The listing builds one solid part. Answer for the finished solid, in the listing's coordinates (mm). Coordinates: 2 decimals unless noted, no trailing zeros. Order: outer loops, then holes, each group sorted by start corner. A loop starts at its lowest first (then second) coordinate and runs counter-clockwise, first axis right, second up. Notation, with made-up numbers: M 24,22 L 41,22 A10 cw 41,35 Z; hole C -6.5,68 d3. An arc over 180 degrees is marked long. One line per item, written item: value. Start each with the question number.
Q1. The part is cut by section A-A on y = 4.45. Give the vertices of the cut face in (x, z), then the cut area to 3 significant figures.
Q2. Straight lines are drawn through the part: line 1 along X through (y, z) = (3.05, -53.5); line 2 along Z through (x, y) = (99, 3); line 3 along X through (y, z) = (5.15, -38). For each, find the intervals that lie inside material, in ascending order. Write a range as [from, to].
Q3. Each of these flat-tipped pins is pushed along its axis until it touches: pin 1 Ø10 at (x, z) = (42, -93) entering from -Y; pin 2 Ø1.7 at (y, z) = (2, -87) entering from -X; pin 3 Ø1 at (y, z) = (1.5, -30) entering from +X. Where does it stop, or does it pass through?
Q4. The part is cut by section B-B on z = -87. Give the vertices of the cut face in (x, y).
```python
from build123d import *

# Parameters (mm, degrees)
SKETCH3_W           = 192
SKETCH3_H           = 135
BOSS_EXTRUDE1_DEPTH = 5.7
SKETCH11_R          = 0.5
CUT_EXTRUDE2_DEPTH  = 33
CUT_EXTRUDE3_DEPTH  = 22


with BuildPart() as part:
    # Sketch3 → Boss-Extrude1 (new body)
    with BuildSketch(Plane(origin=(0, 0, 0), x_dir=(1, 0, 0), z_dir=(0, 1, 0))):
        with Locations((90, 53.5)):
            Rectangle(SKETCH3_W, SKETCH3_H)
    extrude(amount=BOSS_EXTRUDE1_DEPTH)

    # Sketch11 → Cut-Extrude2 (cut)
    with BuildSketch(Plane(origin=(0, 0, 0), x_dir=(1, 0, 0), z_dir=(0, 1, 0))):
        with Locations((99, 53.5)):
            Circle(SKETCH11_R)
        with Locations((154.2, 53.5)):
            Circle(SKETCH11_R)
    extrude(amount=CUT_EXTRUDE2_DEPTH, mode=Mode.SUBTRACT)

    # Sketch12 → Cut-Extrude3 (cut)
    with BuildSketch(Plane(origin=(0, 0, 0), x_dir=(1, 0, 0), z_dir=(0, 1, 0))):
        Polygon((-5.8, 121), (-5.8, 93.9), (0, 93.9), (0, 67.1), (-5.8, 67.1), (-5.8, 39.9), (0, 39.9), (0, 13.1), (-5.8, 13.1), (-5.8, -14), (-9.8, -14), (-9.8, 121), align=None)
        Polygon((189.8, 121), (185.8, 121), (185.8, 93.9), (180, 93.9), (180, 67.1), (185.8, 67.1), (185.8, 39.9), (180, 39.9), (180, 13.1), (185.8, 13.1), (185.8, -14), (189.8, -14), align=None)
    extrude(amount=CUT_EXTRUDE3_DEPTH, mode=Mode.SUBTRACT)


solid = part.part
```
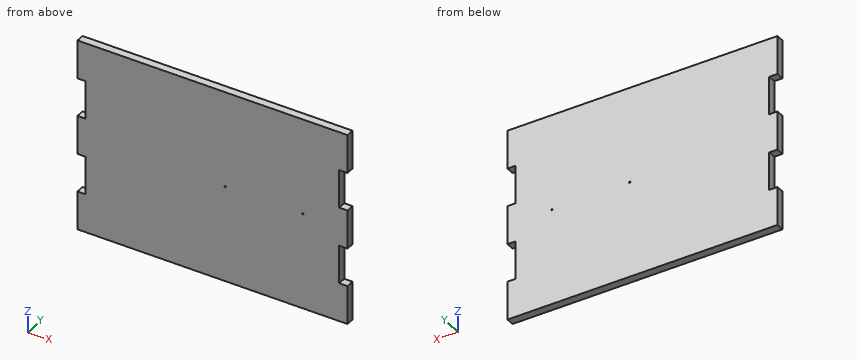
Output:
1. outline: M -5.8,-121 L 185.8,-121 L 185.8,-93.9 L 180,-93.9 L 180,-67.1 L 185.8,-67.1 L 185.8,-39.9 L 180,-39.9 L 180,-13.1 L 185.8,-13.1 L 185.8,14 L -5.8,14 L -5.8,-13.1 L 0,-13.1 L 0,-39.9 L -5.8,-39.9 L -5.8,-67.1 L 0,-67.1 L 0,-93.9 L -5.8,-93.9 Z; hole C 99,-53.5 d1; hole C 154.2,-53.5 d1
1. area: 25,200 mm^2
2. line 1: x = [-5.8, 98.5], [99.5, 153.7], [154.7, 185.8]
2. line 2: z = [-121, -54], [-53, 14]
2. line 3: x = [0, 180]
3. pin 1: stops at y = 0
3. pin 2: stops at x = 0
3. pin 3: stops at x = 180
4. outline: M 0,0 L 180,0 L 180,5.7 L 0,5.7 Z
